Job drawing, mm, ordinate dimensions from the low corner. One solid piece. Round coordinates to 2 decimals unless told otherwise and drop trailing zeros. Loops run counter-clockwise (first coordinate to the right, second up) from the corner with the lowest first, then second, coordinate; pieces in that order, holes last. Notation, with made-up numbers: M 40.5,-17.5 L 59.5,-17.5 A29 cw 59.5,10.5 Z; hole C 67.5,46 d8. An arc over 180 degrees is marked long. Put each result on its own line as item: value. Start each with the question number.
1) Probe line 1 along Z through (x, y) = (22, 2.75); line 2 along Z through (x, y) = (3.5, 0.5) (1 decimal); line 3 along X through (y, z) = (1.8, 39). List the from-to ranges inside material, lowest first.
2) Slice it at C-C on y = 2.45. Give the cut face in (x, z), then the cut area to 3 significant figures.
3) Slice it at A-A on z = 25.4. Give the cut face in (x, y) (1 decimal), then the cut area to 3 significant figures.
4) Drop flat-ended pins along their axis: pin 1 Ø4 at (x, z) = (12.5, 30) entering from -Y; pin 2 Ø1.6 at (y, z) = (2.5, 24) entering from -X. Give the stop position or say it passes through.
5) Slice it at D-D on x = 31. Give the cut face in (y, z) (1 decimal), then the cut area to 3 significant figures.
6) Slice it at B-B on x = 25.4. Give the cut face in (y, z) (1 decimal), then the cut area to 3 significant figures.
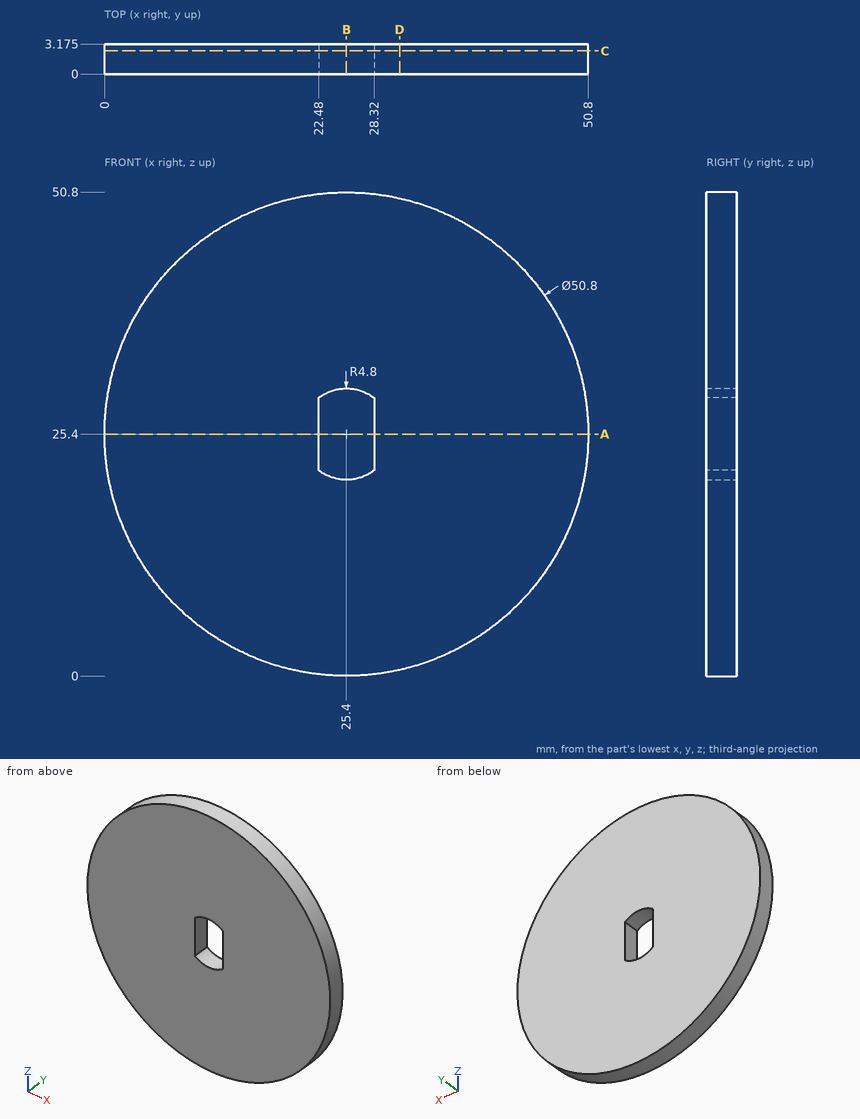
Recorded:
1. line 1: z = 0.23 to 50.57
1. line 2: z = 12.5 to 38.3
1. line 3: x = 3.95 to 46.85
2. outline: C 25.4,25.4 d50.8; hole M 22.48,21.59 A4.8 ccw 28.32,21.59 L 28.32,29.21 A4.8 ccw 22.48,29.21 Z
2. area: 1,970 mm2
3. outline: M 0,0 L 22.5,0 L 22.5,3.2 L 0,3.2 Z; M 28.3,0 L 50.8,0 L 50.8,3.2 L 28.3,3.2 Z
3. area: 143 mm2
4. pin 1: stops at y = 0
4. pin 2: stops at x = 0.01
5. outline: M 0,0.6 L 3.2,0.6 L 3.2,50.2 L 0,50.2 Z
5. area: 157 mm2
6. outline: M 0,0 L 3.2,0 L 3.2,20.6 L 0,20.6 Z; M 0,30.2 L 3.2,30.2 L 3.2,50.8 L 0,50.8 Z
6. area: 131 mm2
